Study the drawing (mm; zero at the part's minimum x, y, z) and answer. A direction names the side the tool comes from. Round coordinates to 2 decimals unless told otherwise and drop trailing zeros. Loops run counter-clockwise (first coordinate to the right, second up) from the corner with the lowest first, then second, coordinate; pieces in that order, holes last. Notation, with made-up numbers: M 51,28.25 L 58,28.25 A36 ccw 58,66.25 Z; hole C 52.5,34 d7. An arc over 180 degrees is marked long. Put each result on its own line as item: value. Start each with the question number.
(1) A straight line is drawn through the part: line 1 (X direction, y = 33.5, z = 40) (3 decimals). Find the intervals that lie inside material, in ascending order.
(2) Section B-B, the plane x = 38 is taken. Determine the outline of the cut face in (y, z) (3 decimals), then the cut area to 3 significant figures.
(3) Which of the six approach directions +Z, -Z, +X, -X, +Y, -Y give full straight-line access (tool end or side, diameter ignored) to the marked faces 1 and 2?
(4) Flat-ended cylindrical pins translate along their axes: P1, Ø12, axis at y = 26, z = 21, coming from the +X side (3 decimals); P2, Ø3, axis at x = 32, z = 108.5, coming from the +Y side (3 decimals). Find the tip coordinate at first contact, or state that the pin passes through.
(5) Section A-A, the plane z = 35.5 is taken. Determine the outline of the cut face in (x, y) (3 decimals), then the cut area to 3 significant figures.
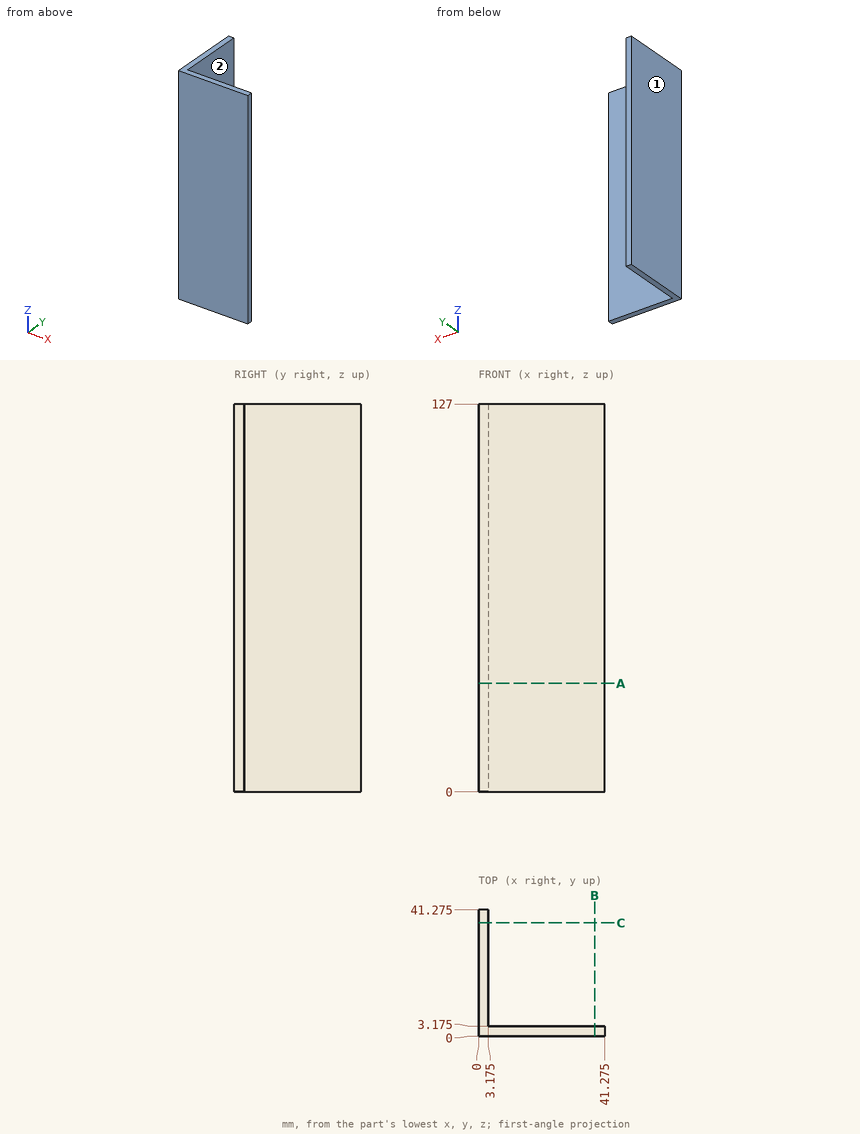
Recorded:
1. line 1: x = 0 to 3.175
2. outline: M 0,0 L 3.175,0 L 3.175,127 L 0,127 Z
2. area: 403 mm²
3. face 1: +Z, -Z, -X, +Y, -Y
3. face 2: +Z, -Z, +X, +Y
4. P1: stops at x = 3.175
4. P2: stops at y = 3.175
5. outline: M 0,0 L 41.275,0 L 41.275,3.175 L 3.175,3.175 L 3.175,41.275 L 0,41.275 Z
5. area: 252 mm²
